For this review, take the finished solid that the model builds, in its own axes (mm). A direction names the side the tool comes from. Coordinates: 2 decimals unless noted, no trailing zeros. Write each loop counter-clockwise with the first axis right and the second up, starting at its lowest first coordinate (ties: lowest second). Pieces come first, ordered by that corner, then holes.
```python
from build123d import *

# Parameters (mm, degrees)
BOSS_EXTRUDE1_DEPTH   = 5
BOSS_EXTRUDE2_DEPTH   = 10
M6X1_0_TAPPED_HOLE1_D = 5
CUT_EXTRUDE1_START    = -10
SKETCH8_R             = 2.5
CUT_EXTRUDE1_DEPTH    = 20


with BuildPart() as part:
    # Sketch1 → Boss-Extrude1 (new, symmetric)
    with BuildSketch(Plane(origin=(0, 0, 0), x_dir=(1, 0, 0), z_dir=(0, 1, 0))):
        with BuildLine():
            Line((-7.5, -0.193392624), (-8.972672616, 28.343633506))
            ThreePointArc((-8.972672616, 28.343633506), (0, 28.575), (8.972672616, 28.343633506))
            Line((8.972672616, 28.343633506), (7.5, -0.193392624))
            ThreePointArc((7.5, -0.193392624), (0, 0), (-7.5, -0.193392624))
        make_face()
    extrude(amount=BOSS_EXTRUDE1_DEPTH, both=True)

    # Sketch2 → Boss-Extrude2 (add, through all)
    with BuildSketch(Plane(origin=(0, 5, 0), x_dir=(1, 0, 0), z_dir=(0, 1, 0))):
        with BuildLine():
            ThreePointArc((-16.404975215, 3.386598502), (0, 4.2875), (16.404975215, 3.386598502))
            ThreePointArc((16.404975215, 3.386598502), (27.439865226, 12.231438943), (18.595024785, 23.266328954))
            ThreePointArc((18.595024785, 23.266328954), (0, 24.2875), (-18.595024785, 23.266328954))
            ThreePointArc((-18.595024785, 23.266328954), (-27.439865226, 12.231438943), (-16.404975215, 3.386598502))
        make_face()
    extrude(amount=-BOSS_EXTRUDE2_DEPTH)

    # M6x1.0 Tapped Hole1 (through all)
    with Locations(Plane(origin=(0, 5, 0), x_dir=(1, 0, 0), z_dir=(0, 1, 0))):
        with Locations((-17.5, 13.326463728), (17.5, 13.326463728)):
            Hole(M6X1_0_TAPPED_HOLE1_D / 2)

    # Sketch8 → Cut-Extrude1 (cut)
    with BuildSketch(Plane.XY.offset(CUT_EXTRUDE1_START)):
        Circle(SKETCH8_R)
    extrude(amount=-CUT_EXTRUDE1_DEPTH, mode=Mode.SUBTRACT)


solid = part.part
```
Q1. Draft analysis for pull direction Z (two halves, no side actions). For faces 1 (the cylindrical face through (20, -0.1, -13.4)), 2 (the flat face through (0, -5, -14)), 3 (the cylindrical face through (0, 0, 0)), state which applies: +Z half, -Z half, draft (parallel to the pull), parting line (faces both ways), or undercut.
Ans:
face 1: undercut
face 2: draft
face 3: +Z half
Q2. Tool access review of faces 4 (the flat face through (-7.61, 0.07, -1.92)), 5 (the flat face through (-8.86, 0.07, -26.17)), 6 (the flat face through (8.864, 0.07, -26.233)): name each direction out of +Z, -Z, +X, -X, +Y, -Y from which nothing blocks a thin tool from reaching the whole face with its end or side.
Ans:
face 4: +Z, +Y, -Y
face 5: -X, +Y, -Y
face 6: +X, +Y, -Y
Q3. Clearance check with flat-ended pins moving along their axes: pin 1 Ø1.5 at (x, y) = (1.5, -1.5) entering from +Z; pin 2 Ø4 at (x, z) = (-17.5, -13.33) entering from -Y; pin 3 Ø1 at (y, z) = (-2.5, -11.5) entering from -X; pin 4 Ø1.5 at (y, z) = (1, -25) entering from +X. State where each tip first meets the part, or that it passes through.
Ans:
pin 1: stops at z = 0.02
pin 2: passes through
pin 3: stops at x = -27.41
pin 4: stops at x = 8.84
Q4. Add section C-C (y = 0). State the section outline as (x, z) points, then the cut area to 3 significant figures.
Ans:
outline: (-18.6, -23.27) arc R169.81 ccw to (-8.75, -24.06) - (-8.97, -28.34) arc R174.1 ccw to (-2.5, -28.56) - (-2.5, -10) - (2.5, -10) - (2.5, -28.56) arc R174.1 ccw to (8.97, -28.34) - (8.75, -24.06) arc R169.81 ccw to (18.6, -23.27) arc R10 ccw to (16.4, -3.39) arc R149.81 cw to (7.72, -4.09) - (7.5, 0.19) arc R145.53 cw to (-7.5, 0.19) - (-7.72, -4.09) arc R149.81 cw to (-16.4, -3.39) arc R10 ccw to start; hole circle Ø5 at (-17.5, -13.33); hole circle Ø5 at (17.5, -13.33)
area: 1,020 mm2
Q5. For probe 1 along X at (y, z) = (-4, -12.25); probe 2 along Y at (x, z) = (0, -25.25); probe 3 along X at (y, z) = (4, -15.5), list the stretches that pass through material, from the lowest coordinate up.
Ans:
probe 1: x = -27.44 to -19.76, -15.24 to 15.24, 19.76 to 27.44
probe 2: y = -5 to -2.5, 2.5 to 5
probe 3: x = -27.26 to -18.74, -16.26 to 16.26, 18.74 to 27.26
Q6. Add section B-B (x = 17.5). State the section outline as (y, z) points.
Ans:
outline: (-5, -23.38) - (5, -23.38) - (5, -15.83) - (-5, -15.83) - close; (-5, -10.83) - (5, -10.83) - (5, -3.33) - (-5, -3.33) - close
Q7. Add section A-A (z = -14). State the section outline as (x, y) points, then the cut area to 3 significant figures.
Ans:
outline: (-27.48, -5) - (-19.91, -5) - (-19.91, 5) - (-27.48, 5) - close; (-15.09, -5) - (15.09, -5) - (15.09, 5) - (-15.09, 5) - close; (19.91, -5) - (27.48, -5) - (27.48, 5) - (19.91, 5) - close; hole circle Ø5 at (0, 0)
area: 434 mm2
Q8. Add section D-D (y = -3.75). State the section outline as (x, z) points, then the cut area to 3 significant figures.
Ans:
outline: (-18.6, -23.27) arc R169.81 ccw to (-8.75, -24.06) - (-8.97, -28.34) arc R174.1 ccw to (8.97, -28.34) - (8.75, -24.06) arc R169.81 ccw to (18.6, -23.27) arc R10 ccw to (16.4, -3.39) arc R149.81 cw to (7.72, -4.09) - (7.5, 0.19) arc R145.53 cw to (-7.5, 0.19) - (-7.72, -4.09) arc R149.81 cw to (-16.4, -3.39) arc R10 ccw to start; hole circle Ø5 at (-17.5, -13.33); hole circle Ø5 at (17.5, -13.33)
area: 1,120 mm2
